Here's the drawing with two shaded views (mm, measured from the low corner). I have some questions. A direction names the side the tool comes from. Round coordinates to 2 decimals unless told otherwise and drop trailing zeros. Order: outer loops, then holes, each group sorted by start corner. A loop starts at its lowest first (then second) coordinate and runs counter-clockwise, first axis right, second up.
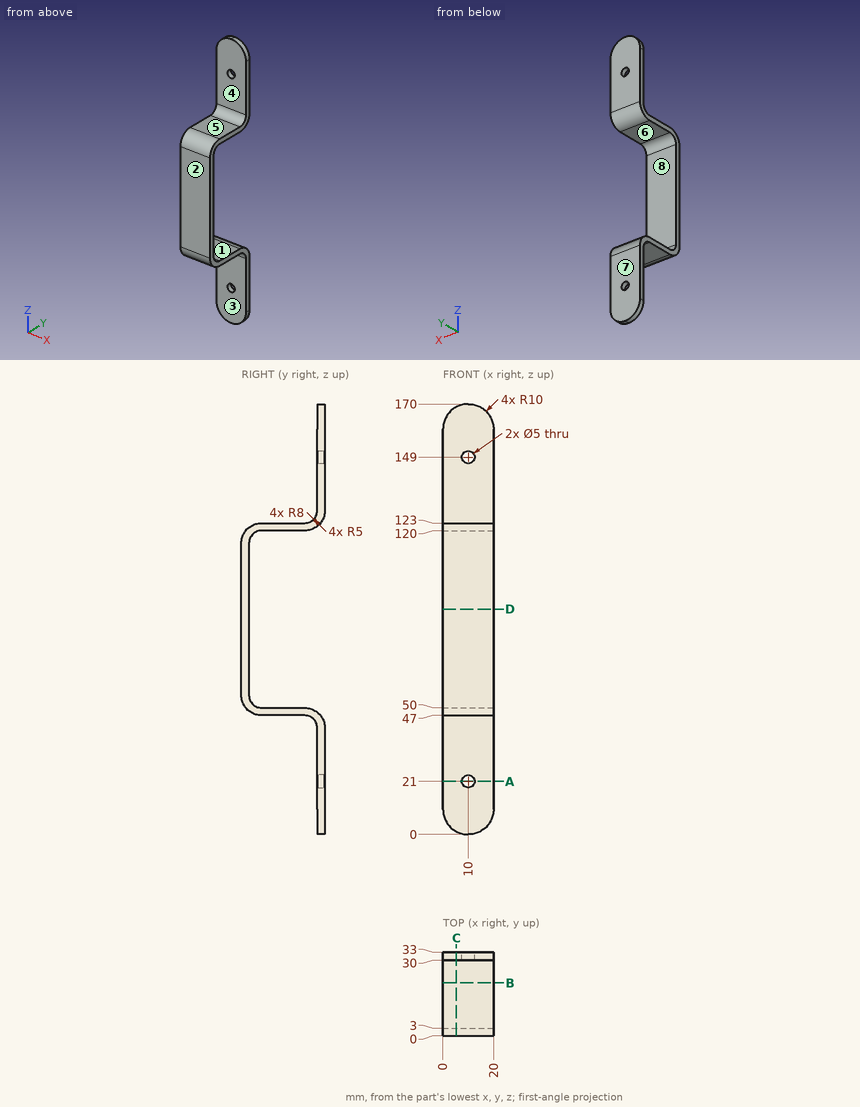
1. I need wall thicknesses on probe 1 along Z at (x, y) = (12.25, 23); probe 2 along X at (y, z) = (31.25, 21); probe 3 along Y at (x, z) = (4, 132.5). Which ranges of each line are inside material? Lowest first, please.
Evaluation:
probe 1: z = 47 to 50, 120 to 123
probe 2: x = 0 to 7.5, 12.5 to 20
probe 3: y = 30 to 33
2. If we section it at B-B, the plane y = 21: Write out the boundary of the cut face in (x, z).
Evaluation:
outline: (0, 47) - (20, 47) - (20, 50) - (0, 50) - close; (0, 120) - (20, 120) - (20, 123) - (0, 123) - close
3. If we section it at D-D, the plane z = 89: Write out the boundary of the cut face in (x, y), and give its area (3 significant figures).
Evaluation:
outline: (0, 0) - (20, 0) - (20, 3) - (0, 3) - close
area: 60.0 mm2
4. If we section it at A-A, the plane z = 21: Write out the boundary of the cut face in (x, y).
Evaluation:
outline: (0, 30) - (7.5, 30) - (7.5, 33) - (0, 33) - close; (12.5, 30) - (20, 30) - (20, 33) - (12.5, 33) - close
5. On a 3-axis mill with a long thin cutter (end or side, diameter ignored), from which of +Z, -Z, +X, -X, +Y, -Y can I reach the whole of each face in a straight line? I mean the marked faces 1, 2, 3 and 4. Say none if no direction works.
Evaluation:
face 1: +X, -X, +Y
face 2: +Z, -Z, +X, -X, -Y
face 3: -Z, +X, -X, -Y
face 4: +Z, +X, -X, -Y
6. If we mould it in two halves opening along Z, with no side actions, what happens to the marked faces 5, 6, 7 and 8? For each: released by +Z, released by -Z, zero draft, split by the parting line, or undercut.
Evaluation:
face 5: released by +Z
face 6: undercut
face 7: zero draft
face 8: undercut
7. I'm going to push flat-ended pins straight in: P1, Ø4, axis at x = 3, y = 21.5, coming from the +Z side; P2, Ø1, axis at x = 13.5, z = 128, coming from the -Y side (3 decimals); P3, Ø1, axis at x = 13.5, z = 107.5, coming from the +Y side; P4, Ø12, axis at y = 22.5, z = 115.5, coming from the -X side. Where does each tip first touch, or does it pass through?
Evaluation:
P1: stops at z = 123
P2: stops at y = 29.975
P3: stops at y = 3
P4: stops at x = 0
8. If we section it at C-C, the plane x = 5.25: Write out the boundary of the cut face in (y, z), and give its area (3 significant figures).
Evaluation:
outline: (0, 55) arc R8 ccw to (8, 47) - (25, 47) arc R5 cw to (30, 42) - (30, 1.2) - (33, 1.2) - (33, 42) arc R8 ccw to (25, 50) - (8, 50) arc R5 cw to (3, 55) - (3, 115) arc R5 cw to (8, 120) - (25, 120) arc R8 ccw to (33, 128) - (33, 168.8) - (30, 168.8) - (30, 128) arc R5 cw to (25, 123) - (8, 123) arc R8 ccw to (0, 115) - close
area: 649 mm2
